Input: part model. Units: mm. Frame: model coordinates. A direction names the side the tool comes from. Coordinates: 2 decimals unless noted, no trailing zeros. Order: outer loops, then holes, each group sorted by start corner. A loop starts at its lowest first (then second) coordinate and runs counter-clockwise, first axis right, second up. Notation, with made-up numbers: M 87.25,-22 L 132.25,-22 A19 cw 132.25,-3 Z; hole C 13.5,-27 d10. An arc over 180 degrees is marked long. One line per item, written item: value.
Autodesk Inventor part; units mm, degrees
ref_plane "YZ Plane" through (0, 0, 0) normal (1, 0, 0) x (0, 1, 0)
ref_plane "XZ Plane" through (0, 0, 0) normal (0, 1, 0) x (-1, 0, 0)
ref_plane "XY Plane" through (0, 0, 0) normal (0, 0, 1) x (1, 0, 0)
sketch "Sketch1" plane through (0, 0, 0) normal (0, 1, 0) x (-1, 0, 0)
  circle A0 centre (0, 0) radius 2
  line L0 (0, 2) -> (22, 2)
  line L1 (22, 2) -> (22, -2)
  line L2 (22, 2) -> (22, 29)
  line L3 (22, 29) -> (62, 29)
  line L4 (22, -2) -> (62, -2)
  line L5 (62, 29) -> (62, -2)
  line L6 (17.9896, 2) -> (17.9896, -2)
  line L7 (62, -2) -> (62, 2)
  line L8 (22, -2) -> (0, -2)
  line L9 (62, 2) -> (84, 2)
  line L10 (62, -2) -> (84, -2)
  circle A1 centre (84, 0) radius 2
  line L11 (66.01, 2) -> (66.01, -2)
  line L12 (66.01, 2) -> (62, 2)
  line L13 (62, -2) -> (66.01, -2)
  line L14 (17.9896, 2) -> (22, 2)
  line L15 (22, -2) -> (17.9896, -2)
  line L16 (66.01, 2) -> (66.01, -2)
  line L17 (62, -2) -> (62, 2)
  line L18 (17.9896, -2) -> (17.9896, 2)
  line L19 (22, 2) -> (22, -2)
  line L20 (66.01, 2) -> (66.01, -2)
  line L21 (62, -2) -> (62, 2)
  line L22 (22, -2) -> (22, 2)
  line L23 (22, -2) -> (22, 2)
  line L24 (22, 2) -> (22, -2)
  line L25 (17.9896, -2) -> (17.9896, 2)
  line L26 (62, 2) -> (66.01, 2)
  line L27 (66.01, -2) -> (62, -2)
  line L28 (22, 2) -> (22, -2)
  line L29 (17.9896, -2) -> (17.9896, 2)
  line L30 (22, 2) -> (17.9896, 2)
  line L31 (22, -2) -> (17.9896, -2)
  line L32 (66.01, 2) -> (62, 2)
  line L33 (62, -2) -> (62, 2)
  line L34 (66.01, -2) -> (62, -2)
  line L35 (66.01, 2) -> (66.01, -2)
  dimension "d0" = 4
  dimension "d8" = 4
  dimension "d9" = 22
  dimension "d13" = 4
  dimension "d16" = 4.01
extrude "Extrusion1" add sketch "Sketch1" against normal blind 7 contours A0 | A1
extrude "Extrusion2" add sketch "Sketch1" along normal blind 5 contours A0 | A0 L0 L6 L8 | L11 L9 A1 L10 | A1
sketch "Sketch2" plane through (0, 5, 0) normal (0, 1, 0) x (1, 0, 0)
  point P0 (0, 0)
extrude "Extrusion3" add sketch "Sketch1" along normal blind 42 contours L0 L1 L8 L6 | L5 L9 L11 L10
extrude "Extrusion4" add sketch "Sketch1" along normal blind 42 contours L2 L3 L5 L4 L1
extrude "Extrusion5" cut sketch "Sketch1" along normal blind 38 contours L2 L3 L5 L4 L1
fillet "Fillet1" radius 2 4 edges at (-66.01, 5, 0) (-66.01, 42, 0) (-17.9896, 42, 0) (-17.9896, 5, 0)
properties part number "recubrimiento de motor"
(1) Draft query along X for faces 5 (the cylindrical face through (-66.58, 5.6, -0.03)), 6 (the cylindrical face through (-18.59, 41.43, -0.03)), 7 (the flat face through (-73, 0, 0)), 8 (the flat face through (0, -7, 0)). Return one class per face: released by +X, released by -X, zero draft, split by the parting line, or undercut.
Data:
face 5: released by -X
face 6: released by +X
face 7: undercut
face 8: zero draft
(2) Access query for faces 1 (the flat face through (-77, 5, 0)), 2 (the cylindrical face through (2, -2, 0)), 3 (the flat face through (-17.99, 23, 0)), 4 (the flat face through (-22, 19, 0)). Directions: +Z, -Z, +X, -X, +Y, -Y. A direction counts if a zero-diameter tool reaches every point of the face in a straight line with its end or side. Return the directions, or none.
Data:
face 1: +Z, -Z, -X, +Y
face 2: -Y
face 3: +Z, -Z, +X, +Y
face 4: +Z, -Z, -Y
(3) Cut plane D-D on x = -9.5. Output: boundary loops of the cut face in (y, z), plus the area to 3 significant figures.
Data:
outline: M 0,-2 L 5,-2 L 5,2 L 0,2 Z
area: 20.0 mm2
(4) First-contact query: pin 1 (3 mm diameter, centred on x = -74.5, z = -0.5, fed in from -Y); pin 2 (1.2 mm diameter, centred on y = 19.5, z = 0.5, fed in from +X); pin 3 (1.2 mm diameter, centred on y = 16, z = -0.5, fed in from -X); pin 4 (6 mm diameter, centred on x = -58, y = 21.5, fed in from +Z). Flat tips, straight axial feed; report the tip coordinate or a pass-through.
Data:
pin 1: stops at y = 0
pin 2: stops at x = -17.99
pin 3: stops at x = -66.01
pin 4: passes through
(5) Cut plane B-B on z = 0. Output: boundary loops of the cut face in (x, y), plus the area to 3 significant figures.
Data:
outline: M -86,-7 L -82,-7 L -82,0 L -62,0 L -62,38 L -22,38 L -22,0 L -2,0 L -2,-7 L 2,-7 L 2,5 L -15.99,5 A2 cw -17.99,7 L -17.99,40 A2 ccw -19.99,42 L -64.01,42 A2 ccw -66.01,40 L -66.01,7 A2 cw -68.01,5 L -86,5 Z
area: 753 mm2
(6) Ray query, line 1 (X direction, y = 10, z = 0); line 2 (Y direction, x = -28, z = 23.5); line 3 (Z direction, x = -21, y = 26). Return the intervals inside material, ascending. Write a range as from..to.
Data:
line 1: x = -66.01..-62, -22..-17.99
line 2: y = 38..42
line 3: z = -2..2
(7) Cut plane C-C on y = 29. Output: boundary loops of the cut face in (x, z).
Data:
outline: M -66.01,-2 L -62,-2 L -62,2 L -66.01,2 Z; M -22,-2 L -17.99,-2 L -17.99,2 L -22,2 Z
(8) Cut plane A-A on y = 2. Output: boundary loops of the cut face in (x, z).
Data:
outline: M -84,-2 L -62,-2 L -62,2 L -84,2 A2 ccw Z; M -22,-2 L 0,-2 A2 ccw 0,2 L -22,2 Z
